Read the model definition and answer for the solid it produces. Units are mm, in the model's axes. Coordinates: 2 decimals unless noted, no trailing zeros. Order: outer loops, then holes, each group sorted by start corner. A loop starts at its lowest first (then second) coordinate and runs counter-clockwise, first axis right, second up.
```python
from build123d import *

# Parameters (mm, degrees)
SKETCH_1_R                   = 100
EXTRUDE_1_DEPTH              = 5
CUT_EXTRUDE_1_REACH          = 143.51
SKETCH_2_R                   = 12.5
SKETCH_2_R_2                 = 4.05
HOLE_WIZARD_M4_1_D           = 3.3
HOLE_WIZARD_M4_1_CSINK_D     = 4.05
HOLE_WIZARD_M4_1_CSINK_ANGLE = 90


with BuildPart() as part:
    # 草图1 → 凸台-拉伸1 (new body)
    with BuildSketch(Plane(origin=(0, 0, 0), x_dir=(1, 0, 0), z_dir=(0, 1, 0))):
        with Locations(Location((0, 0, 0), (0, 0, 270))):
            Circle(SKETCH_1_R)
    extrude(amount=EXTRUDE_1_DEPTH)

    # 草图2 → 切除-拉伸1 (cut, up to next)
    with BuildSketch(Plane(origin=(0, 5, 0), x_dir=(1, 0, 0), z_dir=(0, 1, 0)), mode=Mode.PRIVATE) as cut_extrude_1_sk1:
        with Locations(Location((0, 0, 0), (0, 0, 270))):
            Circle(SKETCH_2_R)
    cut_extrude_1_tool1 = extrude(cut_extrude_1_sk1.sketch, amount=-CUT_EXTRUDE_1_REACH, mode=Mode.PRIVATE) & part.part
    # 草图2 → 切除-拉伸1 (cut, up to next)
    with BuildSketch(Plane(origin=(0, 5, 0), x_dir=(1, 0, 0), z_dir=(0, 1, 0)), mode=Mode.PRIVATE) as cut_extrude_1_sk2:
        with Locations(Location((0, 19.25, 0), (0, 0, 270))):
            Circle(SKETCH_2_R_2)
    cut_extrude_1_tool2 = extrude(cut_extrude_1_sk2.sketch, amount=-CUT_EXTRUDE_1_REACH, mode=Mode.PRIVATE) & part.part
    add(cut_extrude_1_tool1.solids().sort_by_distance((0, 5, 0))[0], mode=Mode.SUBTRACT)
    add(cut_extrude_1_tool2.solids().sort_by_distance((0, 5, -19.25))[0], mode=Mode.SUBTRACT)

    # M4 螺纹孔1 (through all)
    with Locations(Plane(origin=(0, 5, 0), x_dir=(1, 0, 0), z_dir=(0, 1, 0))):
        with Locations((25.11473671, -14.5), (0, 29), (-25.11473671, -14.5)):
            CounterSinkHole(HOLE_WIZARD_M4_1_D / 2, HOLE_WIZARD_M4_1_CSINK_D / 2, counter_sink_angle=HOLE_WIZARD_M4_1_CSINK_ANGLE)


solid = part.part
```
1) A cutting plane is placed at A-A, the plane z = 0. Determine the outline of the cut face in (x, y).
A:
outline: (-100, 0) - (-12.5, 0) - (-12.5, 5) - (-100, 5) - close; (12.5, 0) - (100, 0) - (100, 5) - (12.5, 5) - close
2) Straight lines are drawn through the part: line 1 (X direction, y = 1.3, z = 14.5); line 2 (X direction, y = 0.8, z = -0.5); line 3 (Z direction, x = 3.5, y = 2.6). For each, find the intervals that lie inside material, in ascending order.
A:
line 1: x = -98.94 to -26.76, -23.46 to 23.46, 26.76 to 98.94
line 2: x = -100 to -12.49, 12.49 to 100
line 3: z = -99.94 to -21.29, -17.21 to -12, 12 to 99.94
3) A cutting plane is placed at B-B, the plane y = 3.65. Determine the outline of the cut face in (x, z), and give its area (3 significant figures).
A:
outline: circle Ø200 at (0, 0); hole circle Ø3.3 at (-25.11, 14.5); hole circle Ø25 at (0, 0); hole circle Ø8.1 at (0, -19.25); hole circle Ø3.3 at (0, -29); hole circle Ø3.3 at (25.11, 14.5)
area: 30,800 mm2
4) Flat-ended cylindrical pins translate along their axes: pin 1 Ø3 at (x, z) = (47.5, 16.5) entering from -Y; pin 2 Ø1.5 at (y, z) = (3.5, 5.5) entering from +X; pin 3 Ø3 at (x, y) = (-70, 3) entering from +Z; pin 4 Ø2 at (x, y) = (46.5, 2) entering from -Z. Find the tip coordinate at first contact, or state that the pin passes through.
A:
pin 1: stops at y = 0
pin 2: stops at x = 99.89
pin 3: stops at z = 72.85
pin 4: stops at z = -89.05
5) A cutting plane is placed at D-D, the plane z = 38.5. Determine the outline of the cut face in (x, y).
A:
outline: (-92.29, 0) - (92.29, 0) - (92.29, 5) - (-92.29, 5) - close
6) Determine the mould class of faces 1 (the cylindrical face through (30.04, 2.46, 95.38)), 2 (the cylindrical face through (3.755, 2.535, 11.923)), 3 (the flat face through (-21, 5, -1)) for opening direction Z: pulls with the +Z half, pulls with the -Z half, needs draft (parallel to the pull), parting line crosses it, or undercut.
A:
face 1: parting line crosses it
face 2: undercut
face 3: needs draft
7) A cutting plane is placed at C-C, the plane x = -72. Determine the outline of the cut face in (y, z), and give its area (3 significant figures).
A:
outline: (0, -69.4) - (5, -69.4) - (5, 69.4) - (0, 69.4) - close
area: 694 mm2
